Geometry check sheet. Reference: drawing and pictorial views, mm from the part's lowest x, y, z. A direction names the side the tool comes from. Give positions to 0.01 mm unless a question says otherwise; leave off trailing zeros. Order: outer loops, then holes, each group sorted by start corner. A loop starts at its lowest first (then second) coordinate and runs counter-clockwise, first axis right, second up. Notation, with made-up numbers: M -19,-5.75 L 25,-5.75 A11 ccw 25,7.25 Z; hole C 2,32.5 d2. An arc over 180 degrees is marked long. Answer as CSV lines item,"result".
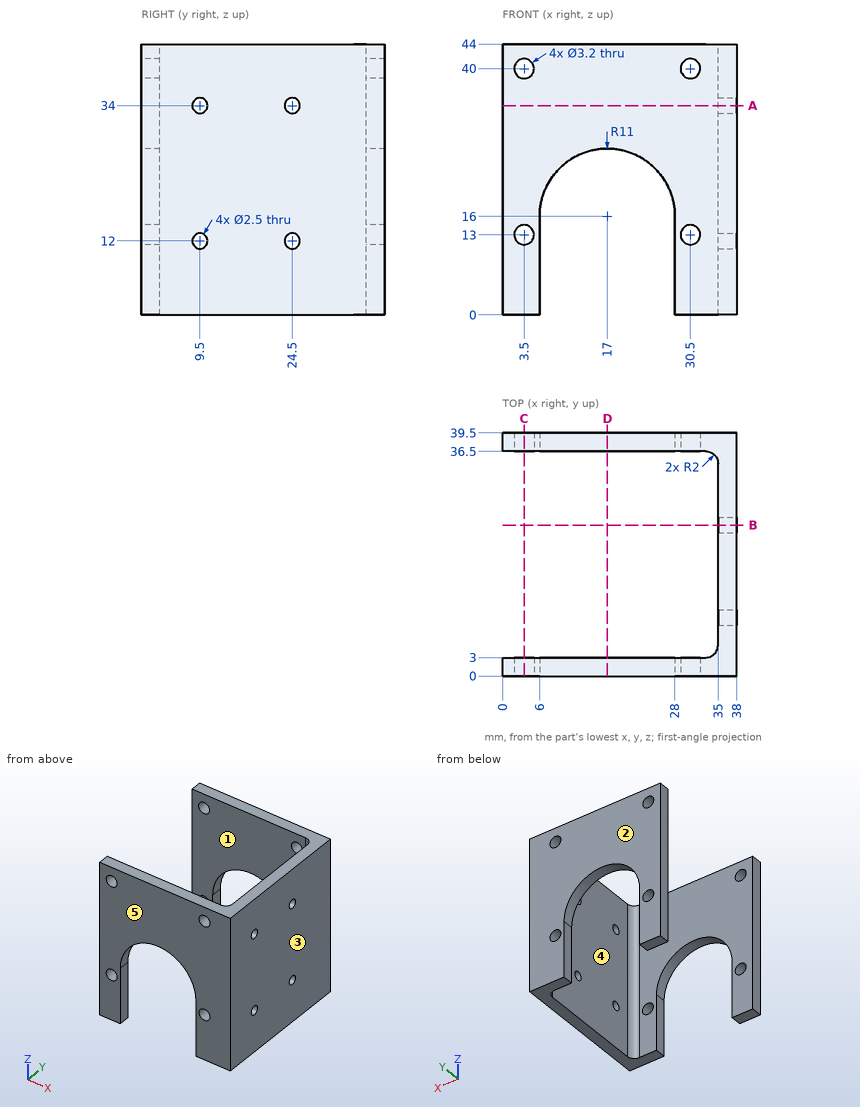
(1) Gauge pin test, flat ends, axial feed: P1, Ø3, axis at y = 24.5, z = 12, coming from the +X side; P2, Ø12, axis at y = 22, z = 37.5, coming from the -X side. Record the tip position at first contact, or that the pin passes through.
The answers:
P1,"stops at x = 38"
P2,"stops at x = 35"
(2) Draft check along Y on the marked faces 1, 2 and 3. Enter one of: +Y half, -Y half, draft (parallel to the pull), parting line (faces both ways), or undercut.
The answers:
face 1,"undercut"
face 2,"+Y half"
face 3,"draft"
(3) Tool access check on the marked faces 4 and 5. Record the directions out of +Z, -Z, +X, -X, +Y, -Y that give a thin tool (end or side, any length) a straight path to the whole face; none if there is none.
The answers:
face 4,"+Z, -Z, -X"
face 5,"+Z, -Z, +X, -X, -Y"
(4) Section check B-B on y = 24.5. Enter the section's corners in (x, z), then the cut area to 3 significant figures.
The answers:
outline,"M 35,0 L 38,0 L 38,10.75 L 35,10.75 Z; M 35,13.25 L 38,13.25 L 38,32.75 L 35,32.75 Z; M 35,35.25 L 38,35.25 L 38,44 L 35,44 Z"
area,"117 mm2"
(5) Material ranges on line 1 (Y direction, x = 36.65, z = 34); line 2 (X direction, y = 1.9, z = 40); line 3 (Z direction, x = 36.1, y = 24.5), recorded low to high.
The answers:
line 1,"y = 0 to 8.25, 10.75 to 23.25, 25.75 to 39.5"
line 2,"x = 0 to 1.9, 5.1 to 28.9, 32.1 to 38"
line 3,"z = 0 to 10.75, 13.25 to 32.75, 35.25 to 44"
(6) Section check C-C on x = 3.5. Enter the section's corners in (y, z).
The answers:
outline,"M 0,0 L 3,0 L 3,11.4 L 0,11.4 Z; M 0,14.6 L 3,14.6 L 3,38.4 L 0,38.4 Z; M 0,41.6 L 3,41.6 L 3,44 L 0,44 Z; M 36.5,0 L 39.5,0 L 39.5,11.4 L 36.5,11.4 Z; M 36.5,14.6 L 39.5,14.6 L 39.5,38.4 L 36.5,38.4 Z; M 36.5,41.6 L 39.5,41.6 L 39.5,44 L 36.5,44 Z"
(7) Section check A-A on z = 34. Enter the section's corners in (x, y), then the cut area to 3 significant figures.
The answers:
outline,"M 0,0 L 38,0 L 38,8.25 L 35,8.25 L 35,5 A2 cw 33,3 L 0,3 Z; M 0,36.5 L 33,36.5 A2 cw 35,34.5 L 35,25.75 L 38,25.75 L 38,39.5 L 0,39.5 Z; M 35,10.75 L 38,10.75 L 38,23.25 L 35,23.25 Z"
area,"315 mm2"
(8) Section check D-D on x = 17. Enter the section's corners in (y, z), then the cut area to 3 significant figures.
The answers:
outline,"M 0,27 L 3,27 L 3,44 L 0,44 Z; M 36.5,27 L 39.5,27 L 39.5,44 L 36.5,44 Z"
area,"102 mm2"
